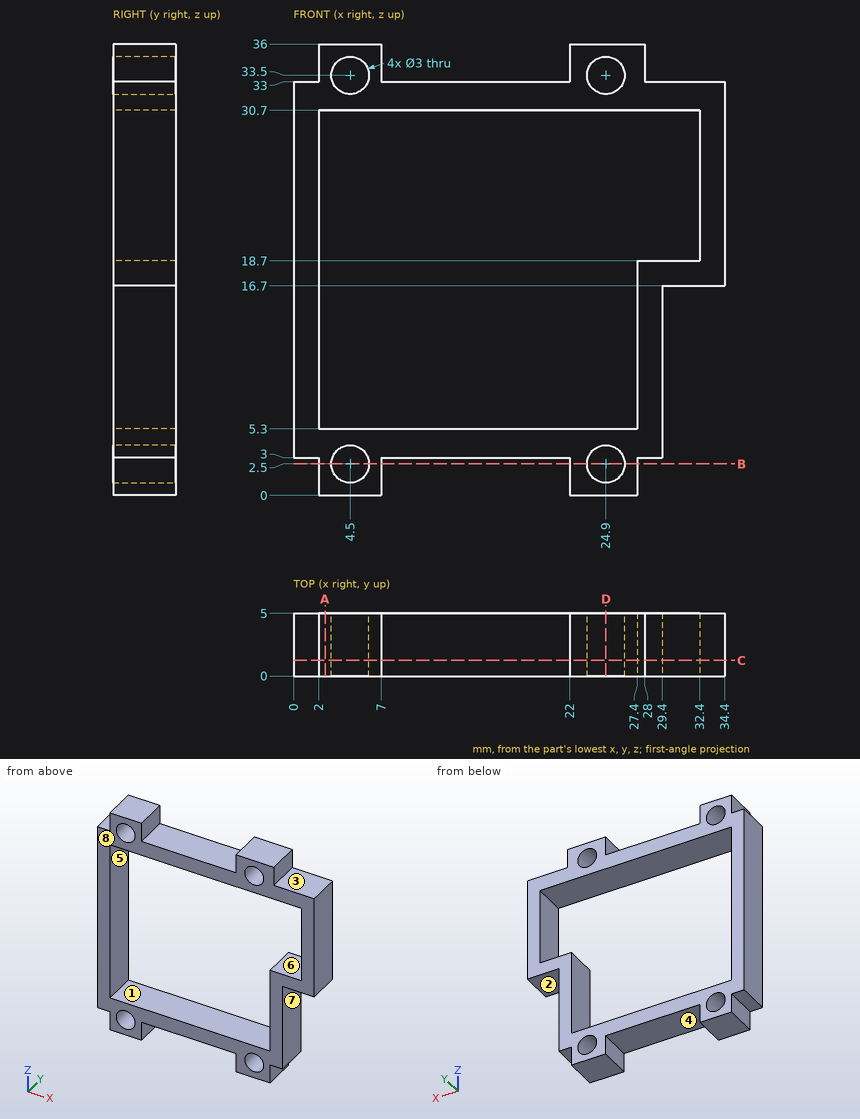
Design review of the part shown in the three views and the two pictorial views. Dimensions are in mm from the part's minimum x, y and z. A direction names the side the tool comes from. Coordinates: 2 decimals unless noted, no trailing zeros. Order: outer loops, then holes, each group sorted by start corner. A loop starts at its lowest first (then second) coordinate and runs counter-clockwise, first axis right, second up. Notation, with made-up numbers: (-7, 27) -> (2, 27) arc R11 ccw to (2, 32) -> close; hole circle Ø7 at (-24.75, 43). An arc over 180 degrees is marked (long way). Use one line per item in the form item = value. Start each with the question number.
(1) Add section C-C on y = 1.25. Give the number of separate pieces and of enclosed holes in the cut face, plus the area to 3 significant figures.
(2) Add section B-B on z = 2.5. State the section outline as (x, y) points.
(3) Insertion check: pin 1 (1.5 mm diameter, centred on y = 1.5, z = 1.5, fed in from +X); pin 2 (1.5 mm diameter, centred on y = 1.5, z = 35, fed in from -X); pin 3 (1.5 mm diameter, centred on x = 17, y = 3, fed in from -Z); pin 4 (2.5 mm diameter, centred on x = 24.9, z = 2.5, fed in from +Y). Each pin has a flat end and moves straight along its axis. Give the tip position at first contact, or say it passes through.
(4) The part is to be moulded in two halves that separate along X. For the marked faces 5, 6, 7 and 8, say which applies: +X half, -X half, draft (parallel to the pull), parting line (faces both ways), or undercut.
(5) Add section A-A on x = 2.5. State the section outline as (y, z) points, plus the area to 3 significant figures.
(6) For the marked faces 1, 2, 3 and 4, list the 3-axis set-ups (+Z, -Z, +X, -X, +Y, -Y) from which the entire face can be reached by the end or side of a thin tool; tool diameter is ignored.
(7) For probe 1 along Z at (x, y) = (8.5, 3); probe 2 along Z at (x, y) = (30, 3.4); probe 3 along X at (y, z) = (2.4, 33.5), list the stretches that pass through material, from the lowest coordinate up.
(8) Add section D-D on x = 24.9. State the section outline as (y, z) points, plus the area to 3 significant figures.
Answer block:
q1.separate_pieces = 1
q1.enclosed_holes = 5
q1.area = 294 mm²
q2.outline = (2, 0) -> (3, 0) -> (3, 5) -> (2, 5) -> close; (6, 0) -> (7, 0) -> (7, 5) -> (6, 5) -> close; (22, 0) -> (23.4, 0) -> (23.4, 5) -> (22, 5) -> close; (26.4, 0) -> (27.4, 0) -> (27.4, 5) -> (26.4, 5) -> close
q3.pin_1 = 27.4
q3.pin_2 = 2
q3.pin_3 = 3
q3.pin_4 = through
q4.face_5 = undercut
q4.face_6 = undercut
q4.face_7 = +X half
q4.face_8 = draft
q5.outline = (0, 0) -> (5, 0) -> (5, 5.3) -> (0, 5.3) -> close; (0, 30.7) -> (5, 30.7) -> (5, 36) -> (0, 36) -> close
q5.area = 53.0 mm²
q6.face_1 = +Y, -Y
q6.face_2 = -Z, +X, +Y, -Y
q6.face_3 = +Z, +X, +Y, -Y
q6.face_4 = -Z, +Y, -Y
q7.probe_1 = 3 to 5.3, 30.7 to 33
q7.probe_2 = 16.7 to 18.7, 30.7 to 33
q7.probe_3 = 2 to 3, 6 to 7, 22 to 23.4, 26.4 to 28
q8.outline = (0, 0) -> (5, 0) -> (5, 1) -> (0, 1) -> close; (0, 4) -> (5, 4) -> (5, 5.3) -> (0, 5.3) -> close; (0, 30.7) -> (5, 30.7) -> (5, 32) -> (0, 32) -> close; (0, 35) -> (5, 35) -> (5, 36) -> (0, 36) -> close
q8.area = 23.0 mm²
